Verification items for the finished model (mm, model axes). A direction names the side the tool comes from. Round coordinates to 2 decimals unless told otherwise and drop trailing zeros. Write each loop counter-clockwise with the first axis right and the second up, starting at its lowest first coordinate (ties: lowest second). Pieces come first, ordered by that corner, then holes. Notation, with made-up numbers: (19, 7.25) -> (65, 7.25) arc R12 cw to (65, 13.25) -> close; hole circle Ø8 at (-22.5, 51). An arc over 180 degrees is marked (long way). Answer as a JSON object with one key per item and string values. Group by question number.
(1) Scan lines: L1, parallel to Y at x = 24.25, z = 533.5; L2, parallel to Y at x = 4, z = 192.5. Record each from-to range of solid material in increasing order. Write a range as from..to.
(2) Sectioned sample at C-C on x = 20. Record the cut outline in (y, z).
(3) Set-up check for faces 1 (the face through (7, 2.29, 912.48)), 2 (the face through (15, 2.54, 453)), 3 (the face through (7, 2, 7)): record each of +Z, -Z, +X, -X, +Y, -Y from which the full face is reachable in a straight line by a thin tool's end or side.
(4) Sectioned sample at A-A on z = 65. Record the cut outline in (x, y) (3 decimals).
(5) Sectioned sample at B-B on y = 11.75. Record the cut outline in (x, z).
(6) Gauge pin test, flat ends, axial feed: pin 1 Ø3 at (x, z) = (17.5, 218) entering from +Y; pin 2 Ø10 at (y, z) = (13.5, 577) entering from +X; pin 3 Ø6 at (x, z) = (6, 452) entering from +Y. Record the tip position at first contact, or that the pin passes through.
Autodesk Inventor part; units mm, degrees
ref_plane "YZ Plane" through (0, 0, 0) normal (1, 0, 0) x (0, 1, 0)
ref_plane "XZ Plane" through (0, 0, 0) normal (0, 1, 0) x (-1, 0, 0)
ref_plane "XY Plane" through (0, 0, 0) normal (0, 0, 1) x (1, 0, 0)
sketch "Sketch1" plane through (0, 0, 0) normal (0, 0, 1) x (1, 0, 0)
  line L0 (0, 0) -> (0, 25.4)
  line L1 (0, 0) -> (25.4, 0)
  line L2 (2.54, 25.4) -> (2.54, 5.715)
  line L3 (5.715, 2.54) -> (25.4, 2.54)
  arc A0 (2.54, 5.715) -> (5.715, 2.54) centre (5.715, 5.715) ccw
  line L4 (0, 25.4) -> (2.54, 25.4)
  line L5 (25.4, 2.54) -> (25.4, 0)
  dimension "d0" = 25.4
  dimension "d1" = 25.4
  dimension "d2" = 2.54
  dimension "d3" = 3.175
extrude "Extrusion1" add sketch "Sketch1" along normal blind 919.48
sketch "Sketch2" plane through (0, 0, 0) normal (0, -1, 0) x (1, 0, 0)
  line L0 (25.4, 0) -> (0, 0)
  line L1 (25.4, 0) -> (25.4, 919.48)
  line L2 (0, 919.48) -> (25.4, 919.48)
  line L3 (0, 919.48) -> (25.4, 894.08)
  line L4 (0, 919.48) -> (60.2005, 919.48) construction
  line L5 (0, 0) -> (25.4, 25.4)
  line L6 (0, 0) -> (85.1364, 0) construction
  dimension "d6" = 45
  dimension "d7" = 45
extrude "Extrusion2" cut sketch "Sketch2" against normal blind 914.4
sketch "Sketch3" plane through (0, 25.4, 919.48) normal (0, 1, 0) x (1, 0, 0)
  line L0 (2.54, 916.94) -> (0, 919.48)
  line L1 (2.54, 916.94) -> (2.54, 2.54)
  line L2 (0, 919.48) -> (2.54, 919.48)
  line L3 (2.54, 916.94) -> (2.54, 919.48)
extrude "Extrusion3" add sketch "Sketch3" against normal blind 2.54
equation "\"d0\" = hubAngleWidth1"
equation "\"d1\" = hubAngleWidth2"
equation "\"d2\" = hubAngleThickness"
equation "\"d3\" = 1.25 * hubAngleThickness"
equation "\"d4\" = hubOuterDiam + 2 * hubAngleThickness"
equation "\"hubOuterDiam\" = 914.4"
equation "\"hubInnerDiam\" = 457.2"
equation "\"hubRingThickness\" = 1.524"
equation "\"hubAngleThickness\" = 2.54"
equation "\"hubAngleWidth1\" = 25.4"
equation "\"hubAngleWidth2\" = 25.4"
properties part number "hubRingJigOuter"
Computed values:
{
 "1": {"L1": "0..2.54", "L2": "0..3.04"},
 "2": {"outline": "(0, 20) -> (2.54, 20) -> (2.54, 899.48) -> (0, 899.48) -> close"},
 "3": {"face 1": "+Z, +X, +Y, -Y", "face 2": "+Z, -Z, +X, +Y", "face 3": "-Z, +X, -Y"},
 "4": {"outline": "(0, 0) -> (25.4, 0) -> (25.4, 2.54) -> (5.715, 2.54) arc R3.175 cw to (2.54, 5.715) -> (2.54, 25.4) -> (0, 25.4) -> close"},
 "5": {"outline": "(0, 0) -> (2.54, 2.54) -> (2.54, 916.94) -> (0, 919.48) -> close"},
 "6": {"pin 1": "y = 2.54", "pin 2": "x = 2.54", "pin 3": "y = 4.07"}
}
